Geometry check sheet. Reference: the model listing, model coordinates, mm. Face numbers are marked on the shaded views. A direction names the side the tool comes from. Give positions to 0.01 mm unless a question says otherwise; leave off trailing zeros. Loops run counter-clockwise (first coordinate to the right, second up) from the corner with the lowest first, then second, coordinate; pieces in that order, holes last. Notation, with made-up numbers: (-30.75, 6.25) - (22.25, 6.25) arc R16 cw to (22.25, 33.25) - close; hole circle Ø4 at (29, 15.25). An arc over 180 degrees is marked (long way). Use a Markdown table: item, result. Add a question column.
1. Cross-section at C-C on x = 0. Count the separate pieces of the cut face and the enclosed holes in it, and give its area (3 significant figures).
2. Set-up check for the marked faces 4 and 5: record each of +Z, -Z, +X, -X, +Y, -Y from which the full face is reachable in a straight line by a thin tool's end or side.
3. Depth check by flat-ended pin: P1, Ø1.5, axis at y = 7, z = 2.5, coming from the +X side; P2, Ø1.5, axis at x = 6.5, y = 4.5, coming from the -Z side; P3, Ø4, axis at x = 0, y = 5, coming from the +Z side. Enter the tip coordinate at first touch or a pass-through.
4. Material ranges on L1, parallel to Y at x = 0, z = 6.7; L2, parallel to X at y = 5.5, z = 0; L3, parallel to Y at x = 0, z = 5.05, recorded low to high.
5. Cross-section at D-D on x = -4.5. Enter the section's corners in (y, z), and give its area (3 significant figures).
6. Draft check along Z on the marked faces 1, 2 and 3. Enter one of: pulls with the +Z half, pulls with the -Z half, needs draft (parallel to the pull), parting line crosses it, or undercut.
7. Cross-section at A-A on z = 0. Enter the section's corners in (x, y), and give its area (3 significant figures).
8. Cross-section at B-B on z = 6.75. Enter the section's corners in (x, y).
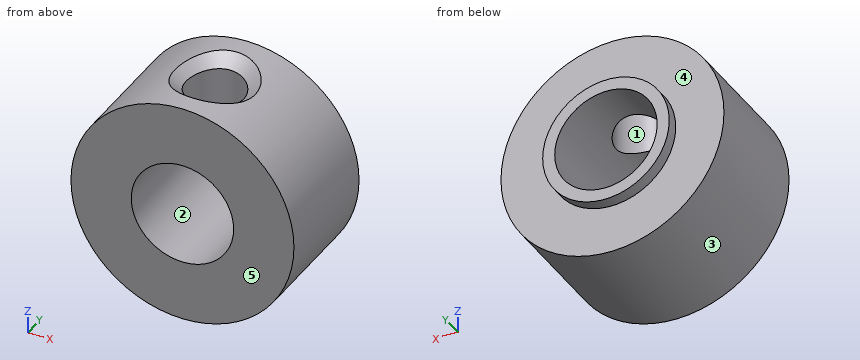
Autodesk Fusion 360 part; units mm, degrees
sketch "Esquisse1" plane through (0, 0, 0) normal (0, 1, 0) x (1, 0, 0)
  circle A0 centre (0, 0) radius 4.25
  circle A1 centre (0, 0) radius 9.25
  circle A2 centre (0, 0) radius 5.25
  dimension "d6" = 8.5
  dimension "d7" = 5
  dimension "d19" = 1
extrude "Extrusion1" add sketch "Esquisse1" along normal blind 10 contours A1 | A2
extrude "Extrusion3" add sketch "Esquisse1" along normal blind 11 contours A2
ref_plane "Plan de construction1" through (0, 6.1987, 9.25) normal (0, 0, 1) x (-1, 0, 0)
sketch "Esquisse2" plane through (0, 6.0312, 9.25) normal (0, 0, 1) x (1, 0, 0)
  line L0 (9.25, 3.9688) -> (-9.25, 3.9688)
  line L1 (9.25, -6.0312) -> (-9.25, -6.0312)
  line L2 (-9.25, 3.9688) -> (9.25, -6.0312) construction
  circle A0 centre (0, -1.0312) radius 2.4
  dimension "d11" = 4.8
extrude "Extrusion2" cut sketch "Esquisse2" against normal blind 9.3
chamfer "Chanfrein1" distance 1 angle 45 2 edges at (2.4, 5, 8.9332) (-2.4, 5, 8.9332)
equation "inner_diam = 8 mm"
equation "insert_len = 4 mm"
equation "margin = 1 mm"
equation "depth = 10 mm"
equation "insert_od = 4.8 mm"
equation "d6 = inner_diam + shaft_tolerance"
equation "d7 = margin + insert_len"
equation "d8 = depth"
equation "d11 = insert_od"
equation "chamfrein = 1 mm"
equation "d13 = -( inner_diam + insert_od * 2 + margin ) / 2"
equation "d15 = chamfrein"
equation "shaft_tolerance = 0.5 mm"
equation "bearing_inner_ring = 1 mm"
equation "spacer_depth = 1 mm"
equation "d19 = bearing_inner_ring"
equation "d20 = depth + spacer_depth"
equation "hex_diam = 24.5 mm"
equation "hex_depth = 8 mm"
equation "wall = 2 mm"
Values found:
| question | item | result |
|---|---|---|
| 1 | separate pieces | 3 |
| 1 | enclosed holes | 0 |
| 1 | area | 77.0 mm2 |
| 2 | face 4 | +Y |
| 2 | face 5 | +Z, -Z, +X, -X, -Y |
| 3 | P1 | stops at x = 9.08 |
| 3 | P2 | stops at z = -7.25 |
| 3 | P3 | stops at z = -3.75 |
| 4 | L1 | y = 0 to 2.6, 7.4 to 10 |
| 4 | L2 | x = -9.25 to -4.25, 4.25 to 9.25 |
| 4 | L3 | y = 0 to 2.6, 7.4 to 11 |
| 5 | outline | (0, -8.08) - (10, -8.08) - (10, -2.7) - (11, -2.7) - (11, 2.7) - (10, 2.7) - (10, 8.08) - (0, 8.08) - close |
| 5 | area | 167 mm2 |
| 6 | face 1 | needs draft |
| 6 | face 2 | undercut |
| 6 | face 3 | parting line crosses it |
| 7 | outline | (-9.25, 0) - (-4.25, 0) - (-4.25, 11) - (-5.25, 11) - (-5.25, 10) - (-9.25, 10) - close; (4.25, 0) - (9.25, 0) - (9.25, 10) - (5.25, 10) - (5.25, 11) - (4.25, 11) - close |
| 7 | area | 102 mm2 |
| 8 | outline | (-6.32, 0) - (6.32, 0) - (6.32, 10) - (-6.32, 10) - close; hole circle Ø4.8 at (0, 5) |
